Autodesk Inventor part; units mm, degrees
ref_plane "YZ Plane" through (0, 0, 0) normal (1, 0, 0) x (0, 1, 0)
ref_plane "XZ Plane" through (0, 0, 0) normal (0, 1, 0) x (-1, 0, 0)
ref_plane "XY Plane" through (0, 0, 0) normal (0, 0, 1) x (1, 0, 0)
sketch "Esquisse1" plane through (0, 0, 0) normal (0, 1, 0) x (-1, 0, 0)
  circle A0 centre (0, 0) radius 1.25
  circle A1 centre (0, 0) radius 2.75
  dimension "d0" = 2.5
  dimension "d1" = 5.5
extrude "Extrusion1" add sketch "Esquisse1" along normal blind 6
sketch "Esquisse2" plane through (0, 6, 0) normal (0, 1, 0) x (1, 0, 0)
  circle A0 centre (0, 0) radius 2.75
  circle A1 centre (0, 0) radius 57.15
  spline S0 degree 3 poles (-57.15, 0) (-60.3141, 7.3699) (-9.2386, 8.3963) (-2.4495, 1.25) knots 0 0 0 0 1 1 1 1
  spline S1 degree 2 poles (-57.15, 0) (-51.1105, -2.5712) (-2.75, 0) knots 0 0 0 1 1 1
  point P0 (-55.0001, 3)
  point P1 (-25, 6)
  point P2 (-51, -1)
  dimension "d4" = 114.3
extrude "Extrusion2" add sketch "Esquisse2" against normal blind 1 contours A0 S1 A1 S0 | A1 S0 picked at (-21.1571, 1.4807)
pattern_circular "Réseau circulaire1" count 2 over 360 about axis through (0, 0, 0) along (0, -1, 0) of "Extrusion2"
properties part number "Helice 4.5x4.5" material "Plastique ABS"
Here's how the part is built. I have some questions about the finished solid (model axes, mm). A direction names the side the tool comes from. Coordinates: 2 decimals unless noted, no trailing zeros. Write each loop counter-clockwise with the first axis right and the second up, starting at its lowest first coordinate (ties: lowest second). Pieces come first, ordered by that corner, then holes.
Item 1: I want a section at B-B on y = 2.75. Write out the boundary of the cut face in (x, z).
Item 2: On a 3-axis mill with a long thin cutter (end or side, diameter ignored), from which of +Z, -Z, +X, -X, +Y, -Y can I reach the whole of each face in a straight line? I mean faces 1 (the flat face through (-1, 0, -1)), 2 (the flat face through (-30, 5, -2)). Say none if no direction works.
Item 3: Will these pins go through, and if not, where does the flat tip stop? pin 1 (6 mm diameter, centred on x = 30, z = 3.5, fed in from -Y); pin 2 (1.5 mm diameter, centred on x = 43, y = 5.5, fed in from -Z); pin 3 (3 mm diameter, centred on y = 1, z = 3.5, fed in from -X).
Item 4: I want a section at A-A on x = 0. Write out the boundary of the cut face in (y, z), and give its area (3 significant figures).
Item 5: If I drill on line 1 (Z direction, x = 0, y = 4.7); line 2 (Y direction, x = -4, z = -1.25); line 3 (X direction, y = 2.5, z = -0.25), over which ranges is the centre line in solid material (lowest first)?
Findings below:
1. outline: circle Ø5.5 at (0, 0); hole circle Ø2.5 at (0, 0)
2. face 1: +Z, -Z, +X, -X, -Y
2. face 2: +Z, -Z, -X, -Y
3. pin 1: stops at y = 5
3. pin 2: stops at z = -1.28
3. pin 3: stops at x = -1.89
4. outline: (0, -2.75) - (6, -2.75) - (6, -1.25) - (0, -1.25) - close; (0, 1.25) - (6, 1.25) - (6, 2.75) - (0, 2.75) - close
4. area: 18.0 mm2
5. line 1: z = -2.75 to -1.25, 1.25 to 2.75
5. line 2: y = 5 to 6
5. line 3: x = -2.74 to -1.22, 1.22 to 2.74
